CAD build for the part. Positions are in the model's coordinates, mm. Face numbers are marked on the shaded views. A direction names the side the tool comes from. Round coordinates to 2 decimals unless told otherwise and drop trailing zeros. Order: outer loops, then holes, each group sorted by start corner. A loop starts at its lowest first (then second) coordinate and runs counter-clockwise, first axis right, second up.
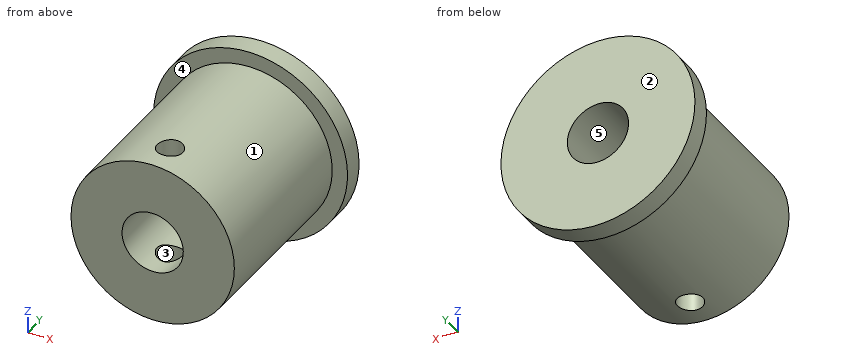
```python
from build123d import *

# Parameters (mm, degrees)
SKETCH1_R           = 4
BOSS_EXTRUDE1_DEPTH = 8.5
SKETCH2_R           = 4.75
BOSS_EXTRUDE2_DEPTH = 1
SKETCH8_R           = 1.5
CUT_EXTRUDE2_DEPTH  = 12.635076278
M1_6_TAPPED_HOLE4_D = 1.25


with BuildPart() as part:
    # Sketch1 → Boss-Extrude1 (new body)
    with BuildSketch(Plane(origin=(0, 0, 0), x_dir=(1, 0, 0), z_dir=(0, 1, 0))):
        with Locations(Location((0, 0, 0), (0, 0, 270))):
            Circle(SKETCH1_R)
    extrude(amount=BOSS_EXTRUDE1_DEPTH)

    # Sketch2 → Boss-Extrude2 (add)
    with BuildSketch(Plane(origin=(0, 8.5, 0), x_dir=(1, 0, 0), z_dir=(0, 1, 0))):
        with Locations(Location((0, 0, 0), (0, 0, 270))):
            Circle(SKETCH2_R)
    extrude(amount=BOSS_EXTRUDE2_DEPTH)

    # Sketch8 → Cut-Extrude2 (cut, through all)
    with BuildSketch(Plane(origin=(0, 9.5, 0), x_dir=(1, 0, 0), z_dir=(0, 1, 0))):
        with Locations(Location((0, 0, 0), (0, 0, 270))):
            Circle(SKETCH8_R)
    extrude(amount=-CUT_EXTRUDE2_DEPTH, mode=Mode.SUBTRACT)

    # M1.6 Tapped Hole4 (through all)
    with Locations(Plane(origin=(0, 0, -5), x_dir=(1, 0, 0), z_dir=(0, 0, -1))):
        with Locations((0, -1.5)):
            Hole(M1_6_TAPPED_HOLE4_D / 2)


solid = part.part
```
1. Cut at D-D, the plane y = 3.25. Write the cut outline in (x, z).
2. Drill centre lines: line 1 (Z direction, x = 0, y = 7); line 2 (Y direction, x = 1, z = 4); line 3 (Z direction, x = 1, y = 1.25). Where is each one in solid material? Low to high.
3. Mould opens along X. For the marked faces 1, 2 and 3 say: released by +X, released by -X, zero draft, split by the parting line, or undercut.
4. Cut at A-A, the plane z = 0. Write the cut outline in (x, y).
5. Cut at C-C, the plane y = 1.5. Write the cut outline in (x, z) (3 decimals), and give its area (3 significant figures).
6. Tool access for the marked faces 4 and 5: list every direction of +Z, -Z, +X, -X, +Y, -Y with a clear straight run to the whole face (end or side of a thin tool).
7. Cut at B-B, the plane x = 0. Write the cut outline in (y, z) (3 decimals), and give its area (4 significant figures).
8. Pin check, flat tips, straight feed: P1, Ø2, axis at y = 3, z = -1.5, coming from the -X side; P2, Ø1.6, axis at x = 0, y = 1.5, coming from the +Z side; P3, Ø5, axis at x = -2, y = 4.5, coming from the -Z side. Stop position of each tip, or through.
Outcome:
1. outline: circle Ø8 at (0, 0); hole circle Ø3 at (0, 0)
2. line 1: z = -4 to -1.5, 1.5 to 4
2. line 2: y = 8.5 to 9.5
2. line 3: z = -3.87 to -1.12, 1.12 to 3.87
3. face 1: split by the parting line
3. face 2: zero draft
3. face 3: undercut
4. outline: (-4.75, 8.5) - (-4, 8.5) - (-4, 0) - (-1.5, 0) - (-1.5, 9.5) - (-4.75, 9.5) - close; (1.5, 0) - (4, 0) - (4, 8.5) - (4.75, 8.5) - (4.75, 9.5) - (1.5, 9.5) - close
5. outline: (-0.625, -3.951) - (-0.625, -1.364) arc R1.5 cw to (-0.625, 1.364) - (-0.625, 3.951) arc R4 ccw to start; (0.625, -3.951) arc R4 ccw to (0.625, 3.951) - (0.625, 1.364) arc R1.5 cw to (0.625, -1.364) - close
5. area: 36.9 mm2
6. face 4: -Y
6. face 5: +Y, -Y
7. outline: (0, -4) - (0.875, -4) - (0.875, -1.5) - (0, -1.5) - close; (0, 1.5) - (0.875, 1.5) - (0.875, 4) - (0, 4) - close; (2.125, -4) - (8.5, -4) - (8.5, -4.75) - (9.5, -4.75) - (9.5, -1.5) - (2.125, -1.5) - close; (2.125, 1.5) - (9.5, 1.5) - (9.5, 4.75) - (8.5, 4.75) - (8.5, 4) - (2.125, 4) - close
7. area: 42.75 mm2
8. P1: stops at x = -3.97
8. P2: stops at z = 4
8. P3: stops at z = -4
